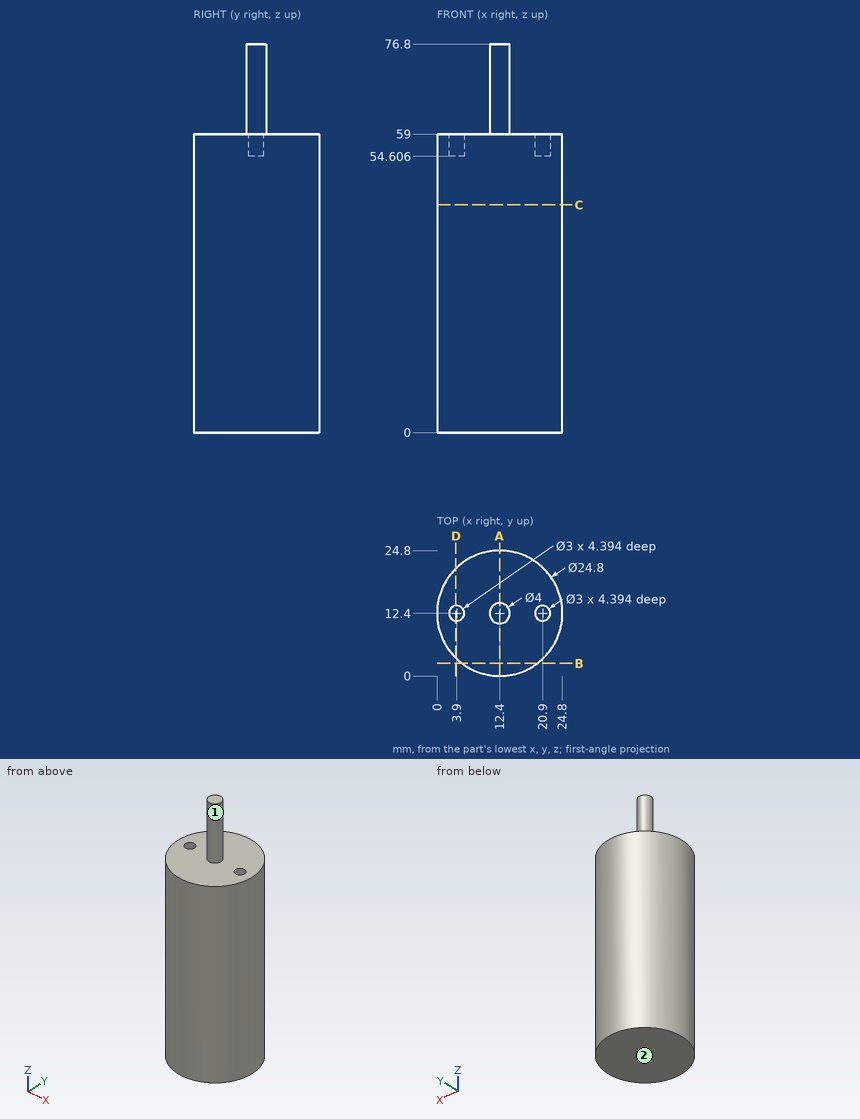
Here's the drawing with two shaded views (mm, measured from the low corner). I have some questions. A direction names the side the tool comes from. Round coordinates to 2 decimals unless told otherwise and drop trailing zeros. Write each loop counter-clockwise with the first axis right and the second up, starting at its lowest first coordinate (ties: lowest second). Pieces come first, ordered by that corner, then holes. Notation, with made-up numbers: M 81.25,-18.75 L 98.25,-18.75 A28 ccw 98.25,4.25 Z; hole C 38.25,-22 d3. An arc over 180 degrees is marked long. Use CSV: the item, a comma, the result in double quotes.
(1) Imagine slicing it at C-C (z = 45). Write out the boundary of the cut face in (x, y).
Check values:
outline,"C 12.4,12.4 d24.8"
(2) Imagine slicing it at D-D (x = 3.75). Write out the boundary of the cut face in (y, z) (1 decimal).
Check values:
outline,"M 3.5,0 L 21.3,0 L 21.3,59 L 13.9,59 L 13.9,54.6 L 10.9,54.6 L 10.9,59 L 3.5,59 Z"
(3) Imagine slicing it at A-A (x = 12.4). Write out the boundary of the cut face in (y, z).
Check values:
outline,"M 0,0 L 24.8,0 L 24.8,59 L 14.4,59 L 14.4,76.8 L 10.4,76.8 L 10.4,59 L 0,59 Z"
(4) Imagine slicing it at B-B (y = 2.5). Write out the boundary of the cut face in (x, z).
Check values:
outline,"M 4.93,0 L 19.87,0 L 19.87,59 L 4.93,59 Z"
(5) On a 3-axis mill with a long thin cutter (end or side, diameter ignored), from which of +Z, -Z, +X, -X, +Y, -Y can I reach the whole of each face in a straight line? I mean the marked faces 1 and 2. Say none if no direction works.
Check values:
face 1,"+Z"
face 2,"-Z, +X, -X, +Y, -Y"
(6) I need wall thicknesses on line 1 along Z through (x, y) = (7, 3); line 2 along Z through (x, y) = (4, 11); line 3 along Y through (x, z) = (20.9, 57.85). Which ranges of each line are inside material? Lowest first, please.
Check values:
line 1,"0 to 59"
line 2,"0 to 54.61"
line 3,"3.37 to 10.9, 13.9 to 21.43"
(7) I'm going to push flat-ended pins straight in: pin 1 (6 mm diameter, centred on y = 8.5, z = 20, fed in from +X); pin 2 (3.5 mm diameter, centred on x = 21, y = 12.5, fed in from +Z); pin 3 (1.8 mm diameter, centred on x = 3.9, y = 12.4, fed in from +Z); pin 4 (10 mm diameter, centred on x = 10.5, y = 11, fed in from -Z). Where does each tip first touch, or does it pass through?
Check values:
pin 1,"x = 24.77"
pin 2,"z = 59"
pin 3,"z = 54.61"
pin 4,"z = 0"
